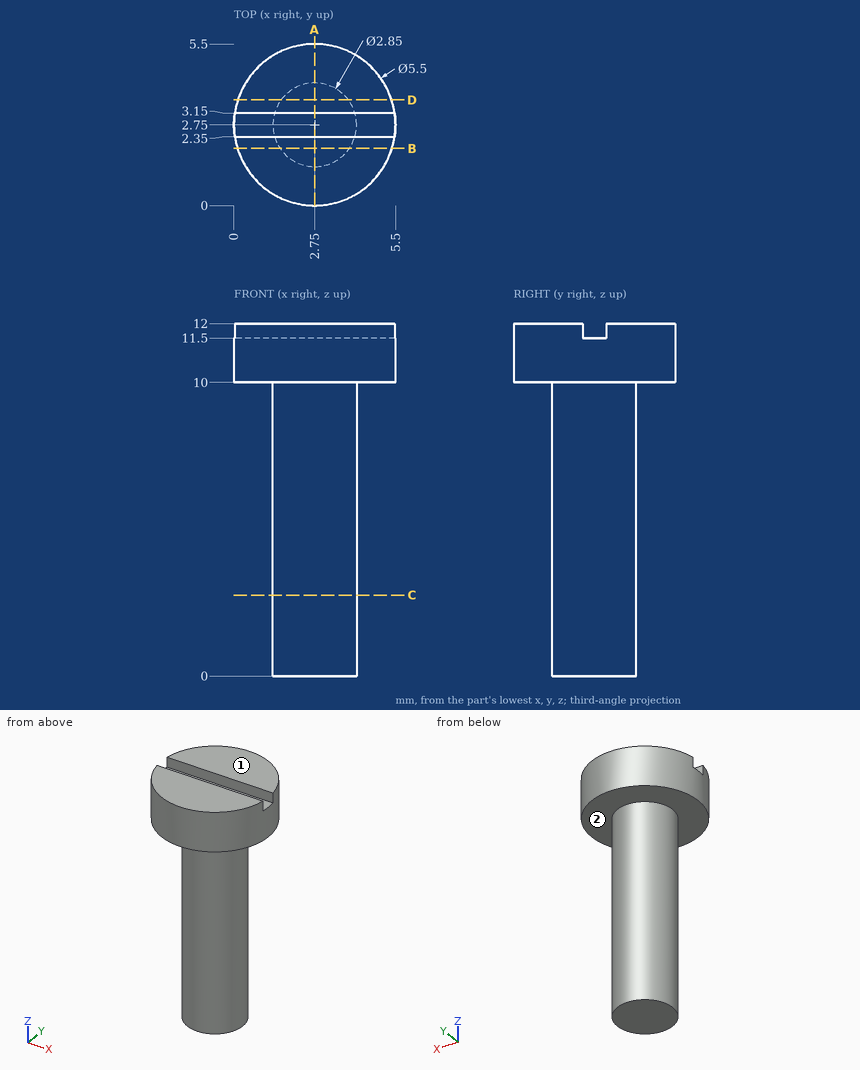
Print and shaded views of the part. All mm, measured from the part's lowest x, y and z. A direction names the side the tool comes from. Coordinates: 2 decimals unless noted, no trailing zeros. Order: outer loops, then holes, each group sorted by start corner. A loop starts at its lowest first (then second) coordinate and runs counter-clockwise, first axis right, second up. Notation, with made-up numbers: (85, 10) -> (123, 10) arc R17 ccw to (123, 14) -> close; hole circle Ø2 at (67.25, 64.25). An arc over 180 degrees is marked (long way). Answer as a JSON object with one key per item and string values. Group by question number.
1) Cut at C-C, the plane z = 2.75. Write the cut outline in (x, y) (3 decimals), then the cut area to 3 significant figures.
2) Cut at A-A, the plane x = 2.75. Write the cut outline in (y, z) (3 decimals).
3) Drill centre lines: L1, parallel to Z at x = 2, y = 0.8; L2, parallel to Y at x = 2.7, z = 3.5; L3, parallel to Z at x = 1.05, y = 2.5. Where is each one in solid material? Low to high.
4) Cut at D-D, the plane y = 3.6. Write the cut outline in (x, z).
5) Flat gauge pins, fed straight in: pin 1 (3 mm diameter, centred on x = 2, y = 1.5, fed in from -Z); pin 2 (1 mm diameter, centred on x = 4.5, y = 1.5, fed in from -Z). Where does each tip first touch, or does it go through?
6) Cut at B-B, the plane y = 1.95. Write the cut outline in (x, z), then the cut area to 3 significant figures.
7) Which spindle directions (+Z, -Z, +X, -X, +Y, -Y) get a long thin tool onto all of the face, cutting with end or side? Do the marked faces 1 and 2. Say none if no direction does.
Check values:
{
 "1": {"outline": "circle Ø2.85 at (2.75, 2.75)", "area": "6.38 mm²"},
 "2": {"outline": "(0, 10) -> (1.325, 10) -> (1.325, 0) -> (4.175, 0) -> (4.175, 10) -> (5.5, 10) -> (5.5, 12) -> (3.15, 12) -> (3.15, 11.5) -> (2.35, 11.5) -> (2.35, 12) -> (0, 12) -> close"},
 "3": {"L1": "z = 10 to 12", "L2": "y = 1.33 to 4.17", "L3": "z = 10 to 11.5"},
 "4": {"outline": "(0.13, 10) -> (1.61, 10) -> (1.61, 0) -> (3.89, 0) -> (3.89, 10) -> (5.37, 10) -> (5.37, 12) -> (0.13, 12) -> close"},
 "5": {"pin 1": "stops at z = 0", "pin 2": "stops at z = 10"},
 "6": {"outline": "(0.12, 10) -> (1.57, 10) -> (1.57, 0) -> (3.93, 0) -> (3.93, 10) -> (5.38, 10) -> (5.38, 12) -> (0.12, 12) -> close", "area": "34.1 mm²"},
 "7": {"face 1": "+Z, +X, -X, +Y, -Y", "face 2": "-Z"}
}
